Read the model definition and answer for the solid it produces. Units are mm, in the model's axes. Round coordinates to 2 decimals unless told otherwise and drop trailing zeros. Write each loop counter-clockwise with the first axis right and the second up, starting at its lowest first coordinate (ties: lowest second). Pieces come first, ordered by that corner, then holes. Notation, with made-up numbers: (81.25, 9.25) -> (101.25, 9.25) arc R20 cw to (101.25, 36.25) -> close; hole circle Ø9 at (-31, 8.25). An arc over 180 degrees is marked (long way). Return JSON: item names as keys, results as strings. Group by question number.
(1) The mould has two halves that part along Z. Classify faces 1 (the flat face through (0, 1, 33)), 2 (the flat face through (-1, 0, -37.8)), 3 (the flat face through (-1, 0, 25)): released by +Z, released by -Z, zero draft, split by the parting line, or undercut.
(2) Straight lines are drawn through the part: line 1 (X direction, y = 0.8, z = 29); line 2 (Y direction, x = 17, z = -26.5). For each, find the intervals that lie inside material, in ascending order.
(3) A cutting plane is placed at B-B on z = -0.5. Give the vertices of the cut face in (x, y).
(4) A cutting plane is placed at A-A on x = 16. Give the vertices of the cut face in (y, z), then the cut area to 3 significant figures.
```python
from build123d import *

# Parameters (mm, degrees)
SKETCH1_W           = 45
SKETCH1_H           = 45
SKETCH1_W_2         = 10
SKETCH1_H_2         = 10
BOSS_EXTRUDE1_DEPTH = 2
SKETCH1_3_W         = 10
SKETCH1_3_H         = 10
SKETCH1_3_H_2       = 45
SKETCH1_3_W_2       = 45
BOSS_EXTRUDE2_DEPTH = 1


with BuildPart() as part:
    # Sketch1 → Boss-Extrude1 (new body)
    # profile 1 of 10: a face of its own
    with BuildSketch(Plane(origin=(0, 0, 0), x_dir=(1, 0, 0), z_dir=(0, 1, 0))):
        Polygon((-37.8, -27.8), (-37.8, -22.5), (-27.8, -22.5), (-27.8, 22.5), (-37.8, 22.5), (-37.8, 27.8), (-27.8, 27.8), (-27.8, 37.8), (-22.5, 37.8), (-22.5, 27.8), (22.5, 27.8), (22.5, 37.8), (27.8, 37.8), (27.8, 27.8), (37.8, 27.8), (37.8, 22.5), (27.8, 22.5), (27.8, -22.5), (37.8, -22.5), (37.8, -27.8), (27.8, -27.8), (27.8, -37.8), (22.5, -37.8), (22.5, -27.8), (-22.5, -27.8), (-22.5, -37.8), (-27.8, -37.8), (-27.8, -27.8), align=None)
        Rectangle(SKETCH1_W, SKETCH1_H, mode=Mode.SUBTRACT)
    # profile 2 of 10: a face of its own
    with BuildSketch(Plane(origin=(0, 0, 0), x_dir=(1, 0, 0), z_dir=(0, 1, 0))):
        with Locations((-32.8, 0)):
            Rectangle(SKETCH1_W_2, SKETCH1_H)
    # profile 3 of 10: a face of its own
    with BuildSketch(Plane(origin=(0, 0, 0), x_dir=(1, 0, 0), z_dir=(0, 1, 0))):
        with Locations((-32.8, -32.8)):
            Rectangle(SKETCH1_W_2, SKETCH1_H_2)
    # profile 4 of 10: a face of its own
    with BuildSketch(Plane(origin=(0, 0, 0), x_dir=(1, 0, 0), z_dir=(0, 1, 0))):
        with Locations((0, -32.8)):
            Rectangle(SKETCH1_W, SKETCH1_H_2)
    # profile 5 of 10: a face of its own
    with BuildSketch(Plane(origin=(0, 0, 0), x_dir=(1, 0, 0), z_dir=(0, 1, 0))):
        with Locations((32.8, -32.8)):
            Rectangle(SKETCH1_W_2, SKETCH1_H_2)
    # profile 6 of 10: a face of its own
    with BuildSketch(Plane(origin=(0, 0, 0), x_dir=(1, 0, 0), z_dir=(0, 1, 0))):
        with Locations((32.8, 0)):
            Rectangle(SKETCH1_W_2, SKETCH1_H)
    # profile 7 of 10: a face of its own
    with BuildSketch(Plane(origin=(0, 0, 0), x_dir=(1, 0, 0), z_dir=(0, 1, 0))):
        Rectangle(SKETCH1_W, SKETCH1_H)
    # profile 8 of 10: a face of its own
    with BuildSketch(Plane(origin=(0, 0, 0), x_dir=(1, 0, 0), z_dir=(0, 1, 0))):
        with Locations((0, 32.8)):
            Rectangle(SKETCH1_W, SKETCH1_H_2)
    # profile 9 of 10: a face of its own
    with BuildSketch(Plane(origin=(0, 0, 0), x_dir=(1, 0, 0), z_dir=(0, 1, 0))):
        with Locations((32.8, 32.8)):
            Rectangle(SKETCH1_W_2, SKETCH1_H_2)
    # profile 10 of 10: a face of its own
    with BuildSketch(Plane(origin=(0, 0, 0), x_dir=(1, 0, 0), z_dir=(0, 1, 0))):
        with Locations((-32.8, 32.8)):
            Rectangle(SKETCH1_W_2, SKETCH1_H_2)
    extrude(amount=-BOSS_EXTRUDE1_DEPTH)

    # Sketch1_3 → Boss-Extrude2 (add)
    with BuildSketch(Plane(origin=(0, 0, 0), x_dir=(1, 0, 0), z_dir=(0, 1, 0))):
        with Locations((-32.8, -32.8)):
            Rectangle(SKETCH1_3_W, SKETCH1_3_H)
        with Locations((-32.8, 0)):
            Rectangle(SKETCH1_3_W, SKETCH1_3_H_2)
        with Locations((-32.8, 32.8)):
            Rectangle(SKETCH1_3_W, SKETCH1_3_H)
        with Locations((0, 32.8)):
            Rectangle(SKETCH1_3_W_2, SKETCH1_3_H)
        with Locations((32.8, 32.8)):
            Rectangle(SKETCH1_3_W, SKETCH1_3_H)
        with Locations((32.8, 0)):
            Rectangle(SKETCH1_3_W, SKETCH1_3_H_2)
        with Locations((32.8, -32.8)):
            Rectangle(SKETCH1_3_W, SKETCH1_3_H)
        with Locations((0, -32.8)):
            Rectangle(SKETCH1_3_W_2, SKETCH1_3_H)
        Rectangle(SKETCH1_3_W_2, SKETCH1_3_H_2)
    extrude(amount=BOSS_EXTRUDE2_DEPTH)


solid = part.part
```
Checks:
{
 "1": {"face 1": "zero draft", "face 2": "released by -Z", "face 3": "undercut"},
 "2": {"line 1": "x = -37.8 to -27.8, -22.5 to 22.5, 27.8 to 37.8", "line 2": "y = -2 to 0"},
 "3": {"outline": "(-37.8, -2) -> (37.8, -2) -> (37.8, 1) -> (27.8, 1) -> (27.8, 0) -> (22.5, 0) -> (22.5, 1) -> (-22.5, 1) -> (-22.5, 0) -> (-27.8, 0) -> (-27.8, 1) -> (-37.8, 1) -> close"},
 "4": {"outline": "(-2, -37.8) -> (1, -37.8) -> (1, -27.8) -> (0, -27.8) -> (0, -22.5) -> (1, -22.5) -> (1, 22.5) -> (0, 22.5) -> (0, 27.8) -> (1, 27.8) -> (1, 37.8) -> (-2, 37.8) -> close", "area": "216 mm^2"}
}
